```python
from build123d import *

# Parameters (mm, degrees)
F0_W     = 22.9125
F0_H     = 12.175
F0_W_2   = 4
F0_H_2   = 3.175
F0_R     = 1.5
F1_DEPTH = 3.175


# Not quite as in the source:
# - a length typed as a fraction of an inch, garbled in the dataset ("3 / 203.2 mm" for 3/8 in), is restored


with BuildPart() as f1:
    # F0 (on Top) → F1 (new body)
    with BuildSketch(Plane.XY):
        with Locations((-5.7368283796, -28.2098180865)):
            Rectangle(F0_W, F0_H)
        with Locations((-12.2805783796, -26.7098180865)):
            Rectangle(F0_W_2, F0_H_2, mode=Mode.SUBTRACT)
        with Locations((-5.7805783796, -26.7098180865)):
            Circle(F0_R, mode=Mode.SUBTRACT)
        with Locations((0.7194216204, -26.7098180865)):
            Rectangle(F0_W_2, F0_H_2, mode=Mode.SUBTRACT)
    extrude(amount=F1_DEPTH)


solid = f1.part
```
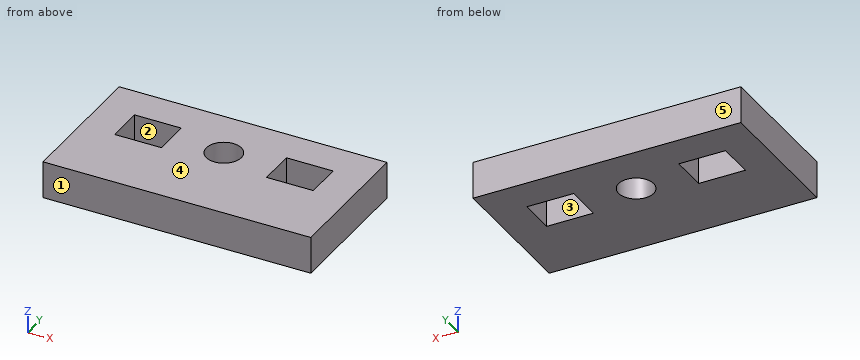
Work out the finished part from the listing and answer in its coordinate system (mm). Face numbers are marked on the shaded views. A direction names the side the tool comes from. Round coordinates to 2 decimals unless told otherwise and drop trailing zeros. Loops run counter-clockwise (first coordinate to the right, second up) from the corner with the lowest first, then second, coordinate; pieces in that order, holes last. Notation, with made-up numbers: (-38.5, 9.5) -> (1.5, 9.5) arc R28 cw to (1.5, 31.5) -> close; hole circle Ø4 at (4, 59). An arc over 180 degrees is marked (long way). Write each question's results on one line, items separated by ' | '. Start each with the question number.
1. Find the intervals of material crossed by probe 1 along X at (y, z) = (-27, 1.4); probe 2 along X at (y, z) = (-27.5, 1.45); probe 3 along Y at (x, z) = (-12.5, 3), in increasing order. Write a range as from..to.
2. For a pull along Y with two mould halves and no side action, classify the marked faces 3, 4 and 5 as +Y half, -Y half, draft (parallel to the pull), parting line (faces both ways), or undercut.
3. Section A-A (x = -5) is taken. Determine the outline of the cut face in (y, z) (3 decimals).
4. Section B-B (z = 2.7) is taken. Determine the outline of the cut face in (x, y), plus the area to 3 significant figures.
5. A tool of negligible diameter and unlimited length cuts with its end or side. For the marked faces 1 and 2, from which of +Z, -Z, +X, -X, +Y, -Y can it reach the whole face along a straight path? Write none if from no direction.
6. Section C-C (x = 2) is taken. Determine the outline of the cut face in (y, z) (3 decimals).
Evaluation:
1) probe 1: x = -17.19..-14.28, -10.28..-7.25, -4.31..-1.28, 2.72..5.72 | probe 2: x = -17.19..-14.28, -10.28..-7.06, -4.51..-1.28, 2.72..5.72 | probe 3: y = -34.3..-28.3, -25.12..-22.12
2) face 3: undercut | face 4: draft | face 5: +Y half
3) outline: (-34.297, 0) -> (-27.991, 0) -> (-27.991, 3.175) -> (-34.297, 3.175) -> close; (-25.429, 0) -> (-22.122, 0) -> (-22.122, 3.175) -> (-25.429, 3.175) -> close
4) outline: (-17.19, -34.3) -> (5.72, -34.3) -> (5.72, -22.12) -> (-17.19, -22.12) -> close; hole (-14.28, -28.3) -> (-10.28, -28.3) -> (-10.28, -25.12) -> (-14.28, -25.12) -> close; hole circle Ø3 at (-5.78, -26.71); hole (-1.28, -28.3) -> (2.72, -28.3) -> (2.72, -25.12) -> (-1.28, -25.12) -> close | area: 246 mm2
5) face 1: +Z, -Z, +X, -X, -Y | face 2: +Z, -Z
6) outline: (-34.297, 0) -> (-28.297, 0) -> (-28.297, 3.175) -> (-34.297, 3.175) -> close; (-25.122, 0) -> (-22.122, 0) -> (-22.122, 3.175) -> (-25.122, 3.175) -> close
